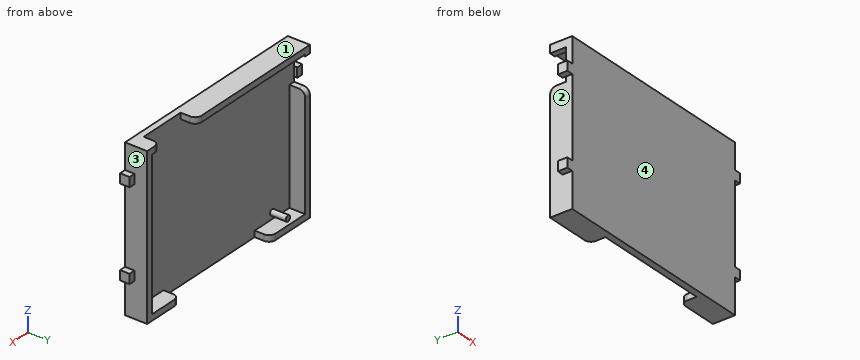
```python
from build123d import *

# Parameters (mm, degrees)
SKETCH_2_W          = 66
SKETCH_2_H          = 50
EXTRUDE_1_DEPTH     = 2
SKETCH_3_W          = 66
SKETCH_3_H          = 50
SKETCH_3_W_2        = 62.2
SKETCH_3_H_2        = 46.2
EXTRUDE_2_DEPTH     = 5
SKETCH_4_W          = 37
SKETCH_4_H          = 6.241197807
CUT_EXTRUDE_1_DEPTH = 5
SKETCH_5_R          = 0.9
EXTRUDE_3_DEPTH     = 5
SKETCH_6_W          = 10
SKETCH_6_H          = 5
CUT_EXTRUDE_2_DEPTH = 5
SKETCH_7_W          = 15
SKETCH_7_H          = 5
CUT_EXTRUDE_3_DEPTH = 5
FILLET_1_R          = 2
SKETCH_8_W          = 3
SKETCH_8_H          = 3
EXTRUDE_4_DEPTH     = 2


with BuildPart() as part:
    # 草图2 → 凸台-拉伸1 (new body)
    with BuildSketch(Plane(origin=(0, 0, 0), x_dir=(1, 0, 0), z_dir=(0, 1, 0))):
        Rectangle(SKETCH_2_W, SKETCH_2_H)
    extrude(amount=EXTRUDE_1_DEPTH)

    # 草图3 → 凸台-拉伸2 (add)
    with BuildSketch(Plane(origin=(0, 2, 0), x_dir=(1, 0, 0), z_dir=(0, 1, 0))):
        Rectangle(SKETCH_3_W, SKETCH_3_H)
        Rectangle(SKETCH_3_W_2, SKETCH_3_H_2, mode=Mode.SUBTRACT)
    extrude(amount=EXTRUDE_2_DEPTH)

    # 草图4 → 切除-拉伸1 (cut)
    with BuildSketch(Plane(origin=(0, 7, 0), x_dir=(1, 0, 0), z_dir=(0, 1, 0))):
        with Locations((1.5, 25.15912339)):
            Rectangle(SKETCH_4_W, SKETCH_4_H)
    extrude(amount=-CUT_EXTRUDE_1_DEPTH, mode=Mode.SUBTRACT)

    # 草图5 → 凸台-拉伸3 (add)
    with BuildSketch(Plane(origin=(0, 2, 0), x_dir=(1, 0, 0), z_dir=(0, 1, 0))):
        with Locations(Location((-24.1, 21.1, 0), (0, 0, 270))):
            Circle(SKETCH_5_R)
    extrude(amount=EXTRUDE_3_DEPTH)

    # 草图6 → 切除-拉伸2 (cut)
    with BuildSketch(Plane.ZY.offset(33)):
        with Locations((17.5, 4.5)):
            Rectangle(SKETCH_6_W, SKETCH_6_H)
    extrude(amount=-CUT_EXTRUDE_2_DEPTH, mode=Mode.SUBTRACT)

    # 草图7 → 切除-拉伸3 (cut)
    with BuildSketch(Plane.XY.offset(25)):
        with Locations((20.5, 4.5)):
            Rectangle(SKETCH_7_W, SKETCH_7_H)
    extrude(amount=-CUT_EXTRUDE_3_DEPTH, mode=Mode.SUBTRACT)

    # 圆角1
    fillet_1_edges = [part.edges().sort_by_distance(p)[0] for p in [
        (13, 7, 24.05),
        (28, 7, 24.05),
        (-17, 7, -24.05),
        (20, 7, -24.05),
        (-32.05, 7, 12.5),
    ]]
    fillet(fillet_1_edges, radius=FILLET_1_R)

    # 草图8 → 凸台-拉伸4 (add)
    with BuildSketch(Plane(origin=(33, 0, 0), x_dir=(0, 0, -1), z_dir=(1, 0, 0))):
        with Locations((-15.5, 1.5)):
            Rectangle(SKETCH_8_W, SKETCH_8_H)
        with Locations((12.5, 1.5)):
            Rectangle(SKETCH_8_W, SKETCH_8_H)
    extrude_4 = extrude(amount=EXTRUDE_4_DEPTH)

    # 镜向1: 凸台-拉伸4 across plane
    add(extrude_4.mirror(Plane(origin=(0, 0, 0), x_dir=(0, 0, 1), z_dir=(1, 0, 0))))


solid = part.part
```
Read the model definition and answer for the solid it produces. Units are mm, in the model's axes. Face numbers are marked on the shaded views. Give positions to 0.01 mm unless a question says otherwise; leave off trailing zeros. Write each loop counter-clockwise with the first axis right and the second up, starting at its lowest first coordinate (ties: lowest second). Pieces come first, ordered by that corner, then holes. Notation, with made-up numbers: (-13, 54.5) -> (14, 54.5) arc R32 ccw to (14, 83.5) -> close; hole circle Ø3 at (-29, 5). An arc over 180 degrees is marked (long way). Answer in a Markdown table with one row per item.
1) Section B-B on z = -3 is taken. Give the vertices of the cut face in (x, y).
Results list:
| item | result |
|---|---|
| outline | (-33, 0) -> (33, 0) -> (33, 7) -> (31.1, 7) -> (31.1, 2) -> (-31.1, 2) -> (-31.1, 7) -> (-33, 7) -> close |
2) Section C-C on x = 5 is taken. Give the vertices of the cut face in (y, z), plus the area to 4 significant figures.
Results list:
| item | result |
|---|---|
| outline | (0, -25) -> (2, -25) -> (2, 23.1) -> (7, 23.1) -> (7, 25) -> (0, 25) -> close |
| area | 109.5 mm^2 |
3) Section A-A on y = 3.75 is taken. Give the vertices of the cut face in (x, z).
Results list:
| item | result |
|---|---|
| outline | (-33, -25) -> (-17, -25) -> (-17, -23.1) -> (-31.1, -23.1) -> (-31.1, 12.5) -> (-33, 12.5) -> close; (-33, 22.5) -> (-31.1, 22.5) -> (-31.1, 23.1) -> (13, 23.1) -> (13, 25) -> (-33, 25) -> close; circle Ø1.8 at (-24.1, -21.1); (20, -25) -> (33, -25) -> (33, 25) -> (28, 25) -> (28, 23.1) -> (31.1, 23.1) -> (31.1, -23.1) -> (20, -23.1) -> close |
4) Each of these flat-tipped pins is pushed along its axis until it touches: pin 1 Ø0.6 at (x, y) = (33.5, 2) entering from -Z; pin 2 Ø1 at (x, y) = (34.5, 2) entering from +Z; pin 3 Ø1.5 at (y, z) = (4.5, 9) entering from -X. Where does it stop, or does it pass through?
Results list:
| item | result |
|---|---|
| pin 1 | z = -14 |
| pin 2 | z = 17 |
| pin 3 | x = -33 |
5) Section D-D on z = -21.1 is taken. Give the vertices of the cut face in (x, y).
Results list:
| item | result |
|---|---|
| outline | (-33, 0) -> (33, 0) -> (33, 7) -> (31.1, 7) -> (31.1, 2) -> (-23.2, 2) -> (-23.2, 7) -> (-25, 7) -> (-25, 2) -> (-31.1, 2) -> (-31.1, 7) -> (-33, 7) -> close |
6) Straight lines are drawn through the part: line 1 (Z direction, x = -20.5, y = 5); line 2 (X direction, y = 3.25, z = -17); line 3 (X direction, y = 1, z = -2). For each, find the intervals that lie inside material, in ascending order. Write a range as [from, to].
Results list:
| item | result |
|---|---|
| line 1 | [-25, -23.1], [23.1, 25] |
| line 2 | [-33, -31.1], [31.1, 33] |
| line 3 | [-33, 33] |
7) Determine the mould class of the marked faces 1, 2, 3 and 4 for opening direction Z: released by +Z, released by -Z, zero draft, split by the parting line, or undercut.
Results list:
| item | result |
|---|---|
| face 1 | released by +Z |
| face 2 | undercut |
| face 3 | undercut |
| face 4 | zero draft |
